Geometry check sheet. Reference: the model listing, model coordinates, mm. A direction names the side the tool comes from. Coordinates: 2 decimals unless noted, no trailing zeros. Loops run counter-clockwise (first coordinate to the right, second up) from the corner with the lowest first, then second, coordinate; pieces in that order, holes last.
from build123d import *

# Parameters (mm, degrees)
EXTRUDE_1_DEPTH          = 1.5
SKETCH_2_W               = 14.8
SKETCH_2_H               = 1.8
EXTRUDE_2_DEPTH          = 5
SKETCH_5_W               = 0.478908464
SKETCH_5_H               = 0.127427029
CUT_EXTRUDE_1_DEPTH      = 0.1
CUT_EXTRUDE_2_DEPTH      = 0.5
CUT_EXTRUDE_2_DEPTH_BACK = 0.5
SKETCH_4_W               = 15.629806388
SKETCH_4_H               = 2.571592952
SKETCH_4_W_2             = 13.8
SKETCH_4_H_2             = 0.8
CUT_EXTRUDE_3_DEPTH      = 117.5
CUT_EXTRUDE_4_DEPTH      = 19.5


with BuildPart() as part:
    # 草图1 → 凸台-拉伸1 (new body)
    with BuildSketch(Plane(origin=(0, 0, 0), x_dir=(1, 0, 0), z_dir=(0, 1, 0))):
        Polygon((-12.4, 6.4), (-9.4, 9.4), (9.4, 9.4), (12.4, 6.4), (12.4, -6.4), (9.4, -9.4), (-9.4, -9.4), (-12.4, -6.4), align=None)
    extrude(amount=EXTRUDE_1_DEPTH)

    # 草图2 → 凸台-拉伸2 (add)
    with BuildSketch(Plane(origin=(0, 1.5, 0), x_dir=(1, 0, 0), z_dir=(0, 1, 0))):
        Rectangle(SKETCH_2_W, SKETCH_2_H)
    extrude(amount=EXTRUDE_2_DEPTH)

    # 草图5 → 切除-拉伸1 (cut)
    with BuildSketch(Plane.XY.offset(0.9)):
        with Locations((-7.4, 3.476334332)):
            Rectangle(SKETCH_5_W, SKETCH_5_H)
    extrude(amount=-CUT_EXTRUDE_1_DEPTH, mode=Mode.SUBTRACT)

    # 草图4 → 切除-拉伸2 (cut, two sides: drawn at the far end of the back side and taken through both)
    with BuildSketch(Plane(origin=(0, 3.412620817, 0), x_dir=(1, 0, 0), z_dir=(0, 1, 0)).offset(-CUT_EXTRUDE_2_DEPTH_BACK)):
        Rectangle(SKETCH_4_W, SKETCH_4_H)
        Rectangle(SKETCH_4_W_2, SKETCH_4_H_2, mode=Mode.SUBTRACT)
    extrude(amount=CUT_EXTRUDE_2_DEPTH + CUT_EXTRUDE_2_DEPTH_BACK, mode=Mode.SUBTRACT)

    # 草图6 → 切除-拉伸3 (cut)
    with BuildSketch(Plane.XY.offset(9.4)):
        Polygon((-6.867040084, 0.488052507), (-6.867040084, 0), (0, 0), (0, 0.859235203), (-7.547096834, 0.859235203), (-7.547096834, 0.488052507), align=None)
        Polygon((0, 0.859235203), (0, 0), (6.867040084, 0), (6.867040084, 0.488052507), (7.547096834, 0.488052507), (7.547096834, 0.859235203), align=None)
    extrude(amount=-CUT_EXTRUDE_3_DEPTH, mode=Mode.SUBTRACT)

    # 草图9 → 切除-拉伸4 (cut)
    with BuildSketch(Plane.XY.offset(9.4)):
        with BuildLine():
            Line((-9.4, 0), (-11.9, 0))
            ThreePointArc((-11.9, 0), (-12.253553391, 0.146446609), (-12.4, 0.5))
            Line((-12.4, 0.5), (-12.4, 1))
            ThreePointArc((-12.4, 1), (-12.253553391, 1.353553391), (-11.9, 1.5))
            Line((-11.9, 1.5), (-13.659182298, 1.5))
            Line((-13.659182298, 1.5), (-13.659182298, -1.631891655))
            Line((-13.659182298, -1.631891655), (14.456410837, -1.631891655))
            Line((14.456410837, -1.631891655), (14.456410837, 1.5))
            Line((14.456410837, 1.5), (11.9, 1.5))
            ThreePointArc((11.9, 1.5), (12.253553391, 1.353553391), (12.4, 1))
            Line((12.4, 1), (12.4, 0.5))
            ThreePointArc((12.4, 0.5), (12.253553391, 0.146446609), (11.9, 0))
            Line((11.9, 0), (9.4, 0))
            Line((9.4, 0), (6.867040084, 0))
            Line((6.867040084, 0), (-6.867040084, 0))
            Line((-6.867040084, 0), (-9.4, 0))
        make_face()
    extrude(amount=-CUT_EXTRUDE_4_DEPTH, mode=Mode.SUBTRACT)


solid = part.part
(1) Access from +Z, -Z, +X, -X, +Y, -Y to the whole of each face (thin tool, end or side, straight path). Record for faces 1 (the flat face through (0, 2, 0.9)), 2 (the flat face through (-7.4, 5, 0)), 3 (the flat face through (9, 0, 0)), 4 (the flat face through (7.4, 5, 0)), 5 (the flat face through (0, 5, -0.9)).
Findings:
face 1: +Z, +X, -X, +Y
face 2: +Z, -Z, -X, +Y
face 3: +Z, -Z, +X, -X, -Y
face 4: +Z, -Z, +X, +Y
face 5: -Z, +X, -X, +Y
(2) Sectioned sample at A-A on z = 3.25. Record the cut outline in (x, y).
Findings:
outline: (-12.4, 0.5) arc R0.5 ccw to (-11.9, 0) - (-6.87, 0) - (-6.87, 0.49) - (-7.55, 0.49) - (-7.55, 0.86) - (7.55, 0.86) - (7.55, 0.49) - (6.87, 0.49) - (6.87, 0) - (11.9, 0) arc R0.5 ccw to (12.4, 0.5) - (12.4, 1) arc R0.5 ccw to (11.9, 1.5) - (-11.9, 1.5) arc R0.5 ccw to (-12.4, 1) - close
(3) Gauge pin test, flat ends, axial feed: pin 1 Ø0.5 at (x, z) = (7.5, -2) entering from +Y; pin 2 Ø7.5 at (x, z) = (-0.5, 4.5) entering from -Y; pin 3 Ø0.7 at (y, z) = (2, 0) entering from +X. Record the tip position at first contact, or that the pin passes through.
Findings:
pin 1: stops at y = 1.5
pin 2: stops at y = 0.86
pin 3: stops at x = 7.4
(4) Scan lines: L1, parallel to X at y = 0.75, z = -5.5; L2, parallel to Y at x = 4.5, z = -0.5; L3, parallel to Y at x = -7.75, z = 6.75. Record each from-to range of solid material in increasing order.
Findings:
L1: x = -12.4 to -7.55, 7.55 to 12.4
L2: y = 0.86 to 2.91, 3.91 to 6.5
L3: y = 0 to 1.5
(5) Sectioned sample at D-D on y = 3.5. Record the cut outline in (x, z).
Findings:
outline: (-6.9, -0.4) - (6.9, -0.4) - (6.9, 0.4) - (-6.9, 0.4) - close
(6) Sectioned sample at B-B on x = 3.75. Record the cut outline in (y, z), and give its area (3 significant figures).
Findings:
outline: (0.86, -9.4) - (1.5, -9.4) - (1.5, -0.9) - (2.91, -0.9) - (2.91, -0.4) - (3.91, -0.4) - (3.91, -0.9) - (6.5, -0.9) - (6.5, 0.9) - (3.91, 0.9) - (3.91, 0.4) - (2.91, 0.4) - (2.91, 0.9) - (1.5, 0.9) - (1.5, 9.4) - (0.86, 9.4) - close
area: 20.0 mm2
(7) Sectioned sample at C-C on y = 2. Record the cut outline in (x, z).
Findings:
outline: (-7.4, -0.9) - (7.4, -0.9) - (7.4, 0.9) - (-7.4, 0.9) - close
(8) Draft check along Y on faces 6 (the flat face through (-0.1, 3.4, -0.4)), 7 (the flat face through (-9, 0, 0)), 8 (the flat face through (0, 6.5, 0)), 9 (the flat face through (0, 2, -0.9)). Enter one of: +Y half, -Y half, draft (parallel to the pull), parting line (faces both ways), or undercut.
Findings:
face 6: undercut
face 7: -Y half
face 8: +Y half
face 9: draft
